from build123d import *

# Parameters (mm, degrees)
SKETCH1_W                      = 152.4
SKETCH1_H                      = 101.6
BASE_FLANGE1_DEPTH             = 1.29032
EDGE_FLANGE1_STRIP_W           = 5.85978
EDGE_FLANGE1_STRIP_H           = 1.29032
EDGE_FLANGE1_STRIP_CUT_DEPTH   = 101.6
EDGE_FLANGE1_STRIP_2_W         = 5.85978
EDGE_FLANGE1_STRIP_2_H         = 1.29032
EDGE_FLANGE1_STRIP_CUT_2_DEPTH = 101.6
EDGE_FLANGE1_DEPTH             = 101.6
EDGE_FLANGE1_BEND_DEPTH        = 101.6
M3X0_5_TAPPED_HOLE1_REACH      = 172.432
M3X0_5_TAPPED_HOLE1_BORE_R     = 1.5
BREAK_CORNER1_START            = -77.68082
BREAK_CORNER1_DEPTH            = 155.36164
CUT_THICKEN1_START             = 48.26
CUT_THICKEN1_OUTLINE_W         = 0.127
CUT_THICKEN1_OUTLINE_H         = 1.29032
CUT_THICKEN1_DEPTH             = 2.54
CUT_THICKEN2_START             = 48.26
CUT_THICKEN2_OUTLINE_W         = 0.127
CUT_THICKEN2_OUTLINE_H         = 1.29032
CUT_THICKEN2_DEPTH             = 2.54
MIRROR7_START                  = 48.26
MIRROR7_COPY_1_SKETCH_W        = 0.127
MIRROR7_COPY_1_SKETCH_H        = 1.29032
MIRROR7_COPY_1_DEPTH           = 2.54
MIRROR7_COPY_2_SKETCH_W        = 0.127
MIRROR7_COPY_2_SKETCH_H        = 1.29032
MIRROR7_COPY_2_DEPTH           = 2.54
MOVE_FACE1_BY                  = 1.27
MOVE_FACE1_2_BY                = 1.27
MOVE_FACE1_3_BY                = 1.27
MOVE_FACE1_4_BY                = 1.27
EDGE_FLANGE2_STRIP_W           = 5.66928
EDGE_FLANGE2_STRIP_H           = 1.29032
EDGE_FLANGE2_STRIP_CUT_DEPTH   = 2.54
EDGE_FLANGE2_STRIP_2_W         = 5.66928
EDGE_FLANGE2_STRIP_2_H         = 1.29032
EDGE_FLANGE2_STRIP_CUT_2_DEPTH = 2.54
EDGE_FLANGE2_STRIP_3_W         = 5.66928
EDGE_FLANGE2_STRIP_3_H         = 1.29032
EDGE_FLANGE2_STRIP_CUT_3_DEPTH = 2.54
EDGE_FLANGE2_STRIP_4_W         = 5.66928
EDGE_FLANGE2_STRIP_4_H         = 1.29032
EDGE_FLANGE2_STRIP_CUT_4_DEPTH = 2.54
EDGE_FLANGE2_DEPTH             = 2.54
EDGE_FLANGE2_BEND_DEPTH        = 2.54
EDGE_FLANGE2_BEND_2_DEPTH      = 2.54
EDGE_FLANGE2_BEND_3_DEPTH      = 2.54


# Read off the part's stored shape, not the designer's step: Break-Corner1, Cut-Thicken1, Cut-Thicken2
# Sheet-metal steps are written as plain solids
with BuildPart() as part:
    # Sketch1 → Base-Flange1 (new body)
    with BuildSketch(Plane.XY):
        Rectangle(SKETCH1_W, SKETCH1_H)
    extrude(amount=-BASE_FLANGE1_DEPTH)

    # Edge-Flange1 strip (across the edge) → Edge-Flange1 strip cut (cut)
    with BuildSketch(Plane(origin=(-76.3905, -50.8, -1.29032), x_dir=(1, 0, 0), z_dir=(0, 1, 0))):
        with Locations((-2.67589, -0.64516)):
            Rectangle(EDGE_FLANGE1_STRIP_W, EDGE_FLANGE1_STRIP_H)
    extrude(amount=EDGE_FLANGE1_STRIP_CUT_DEPTH, mode=Mode.SUBTRACT)

    # Edge-Flange1 strip 2 (across the edge) → Edge-Flange1 strip cut 2 (cut)
    with BuildSketch(Plane(origin=(76.3905, 50.8, -1.29032), x_dir=(-1, 0, 0), z_dir=(0, -1, 0))):
        with Locations((-2.67589, -0.64516)):
            Rectangle(EDGE_FLANGE1_STRIP_2_W, EDGE_FLANGE1_STRIP_2_H)
    extrude(amount=EDGE_FLANGE1_STRIP_CUT_2_DEPTH, mode=Mode.SUBTRACT)

    # Edge-Flange1 section (across the edge) → Edge-Flange1 (add)
    with BuildSketch(Plane(origin=(-76.3905, -50.8, -1.29032), x_dir=(1, 0, 0), z_dir=(0, 1, 0))):
        with BuildLine():
            Line((-1.29032, 0.254), (-1.29032, 46.96968))
            Line((-1.29032, 46.96968), (0, 46.96968))
            Line((0, 46.96968), (0, 0.254))
            ThreePointArc((0, 0.254), (0.074394878, 0.074394878), (0.254, 0))
            Line((0.254, 0), (0.254, -1.29032))
            ThreePointArc((0.254, -1.29032), (-0.837999144, -0.837999144), (-1.29032, 0.254))
        make_face()
    extrude(amount=EDGE_FLANGE1_DEPTH)

    # Edge-Flange1 section 2 (across the edge) → Edge-Flange1 bend (add)
    with BuildSketch(Plane(origin=(76.3905, 50.8, -1.29032), x_dir=(-1, 0, 0), z_dir=(0, -1, 0))):
        with BuildLine():
            Line((-1.29032, 0.254), (-1.29032, 46.96968))
            Line((-1.29032, 46.96968), (0, 46.96968))
            Line((0, 46.96968), (0, 0.254))
            ThreePointArc((0, 0.254), (0.074394878, 0.074394878), (0.254, 0))
            Line((0.254, 0), (0.254, -1.29032))
            ThreePointArc((0.254, -1.29032), (-0.837999144, -0.837999144), (-1.29032, 0.254))
        make_face()
    extrude(amount=EDGE_FLANGE1_BEND_DEPTH)

    # M3x0.5 Tapped Hole1 bore → M3x0.5 Tapped Hole1 (cut, up to next)
    with BuildSketch(Plane.ZY.offset(77.68082), mode=Mode.PRIVATE) as m3x0_5_tapped_hole1_sk1:
        with Locations((-44.7675, 0)):
            Circle(M3X0_5_TAPPED_HOLE1_BORE_R)
    m3x0_5_tapped_hole1_tool1 = extrude(m3x0_5_tapped_hole1_sk1.sketch, amount=-M3X0_5_TAPPED_HOLE1_REACH, mode=Mode.PRIVATE) & part.part
    m3x0_5_tapped_hole1 = m3x0_5_tapped_hole1_tool1.solids().sort_by_distance((-77.68082, 0, -44.7675))[0]
    add(m3x0_5_tapped_hole1, mode=Mode.SUBTRACT)

    # Mirror1: M3x0.5 Tapped Hole1 across plane
    add(m3x0_5_tapped_hole1.mirror(Plane(origin=(0, 0, 0), x_dir=(0, 0, 1), z_dir=(1, 0, 0))), mode=Mode.SUBTRACT)

    # Break-Corner1 outline → Break-Corner1 (cut)
    with BuildSketch(Plane.YZ.offset(BREAK_CORNER1_START)):
        with BuildLine():
            Line((50.8, -48.26), (50.8, -48.006))
            ThreePointArc((50.8, -48.006), (50.725605122, -48.185605122), (50.546, -48.26))
            Line((50.546, -48.26), (50.8, -48.26))
        make_face()
        with BuildLine():
            Line((-50.8, -48.26), (-50.546, -48.26))
            ThreePointArc((-50.546, -48.26), (-50.725605122, -48.185605122), (-50.8, -48.006))
            Line((-50.8, -48.006), (-50.8, -48.26))
        make_face()
    extrude(amount=BREAK_CORNER1_DEPTH, mode=Mode.SUBTRACT)

    # Cut-Thicken1 outline → Cut-Thicken1 (cut)
    with BuildSketch(Plane(origin=(0, 0, 0), x_dir=(1, 0, 0), z_dir=(0, 1, 0)).offset(CUT_THICKEN1_START)):
        with Locations((36.97732, 0.64516)):
            Rectangle(CUT_THICKEN1_OUTLINE_W, CUT_THICKEN1_OUTLINE_H)
    cut_thicken1 = extrude(amount=CUT_THICKEN1_DEPTH, mode=Mode.SUBTRACT)

    # Cut-Thicken2 outline → Cut-Thicken2 (cut)
    with BuildSketch(Plane(origin=(0, 0, 0), x_dir=(1, 0, 0), z_dir=(0, 1, 0)).offset(CUT_THICKEN2_START)):
        with Locations((39.64432, 0.64516)):
            Rectangle(CUT_THICKEN2_OUTLINE_W, CUT_THICKEN2_OUTLINE_H)
    cut_thicken2 = extrude(amount=CUT_THICKEN2_DEPTH, mode=Mode.SUBTRACT)

    # Mirror6: Cut-Thicken1, Cut-Thicken2 across plane
    add(cut_thicken1.mirror(Plane(origin=(0, 0, 0), x_dir=(0, 0, 1), z_dir=(1, 0, 0))), mode=Mode.SUBTRACT)
    add(cut_thicken2.mirror(Plane(origin=(0, 0, 0), x_dir=(0, 0, 1), z_dir=(1, 0, 0))), mode=Mode.SUBTRACT)

    # Mirror7: Cut-Thicken1, Cut-Thicken2 across plane
    add(cut_thicken1.mirror(Plane.ZX), mode=Mode.SUBTRACT)
    add(cut_thicken2.mirror(Plane.ZX), mode=Mode.SUBTRACT)

    # Mirror7 copy 1 sketch → Mirror7 copy 1 (cut)
    with BuildSketch(Plane(origin=(0, 0, 0), x_dir=(-1, 0, 0), z_dir=(0, -1, 0)).offset(MIRROR7_START)):
        with Locations((36.97732, 0.64516)):
            Rectangle(MIRROR7_COPY_1_SKETCH_W, MIRROR7_COPY_1_SKETCH_H)
    extrude(amount=MIRROR7_COPY_1_DEPTH, mode=Mode.SUBTRACT)

    # Mirror7 copy 2 sketch → Mirror7 copy 2 (cut)
    with BuildSketch(Plane(origin=(0, 0, 0), x_dir=(-1, 0, 0), z_dir=(0, -1, 0)).offset(MIRROR7_START)):
        with Locations((39.64432, 0.64516)):
            Rectangle(MIRROR7_COPY_2_SKETCH_W, MIRROR7_COPY_2_SKETCH_H)
    extrude(amount=MIRROR7_COPY_2_DEPTH, mode=Mode.SUBTRACT)

    # Move Face1: a face moved inward by 1.27
    extrude(part.faces().sort_by_distance((-38.31082, -50.8, -0.64516))[0], amount=MOVE_FACE1_BY, dir=(0, 1, 0), mode=Mode.SUBTRACT)

    # Move Face1 2: a face moved inward by 1.27
    extrude(part.faces().sort_by_distance((38.31082, -50.8, -0.64516))[0], amount=MOVE_FACE1_2_BY, dir=(0, 1, 0), mode=Mode.SUBTRACT)

    # Move Face1 3: a face moved inward by 1.27
    extrude(part.faces().sort_by_distance((-38.31082, 50.8, -0.64516))[0], amount=MOVE_FACE1_3_BY, dir=(0, -1, 0), mode=Mode.SUBTRACT)

    # Move Face1 4: a face moved inward by 1.27
    extrude(part.faces().sort_by_distance((38.31082, 50.8, -0.64516))[0], amount=MOVE_FACE1_4_BY, dir=(0, -1, 0), mode=Mode.SUBTRACT)

    # Edge-Flange2 strip (across the edge) → Edge-Flange2 strip cut (cut)
    with BuildSketch(Plane(origin=(37.04082, 49.53, -1.29032), x_dir=(0, -1, 0), z_dir=(1, 0, 0))):
        with Locations((-1.29032, -0.64516)):
            Rectangle(EDGE_FLANGE2_STRIP_W, EDGE_FLANGE2_STRIP_H)
    extrude(amount=EDGE_FLANGE2_STRIP_CUT_DEPTH, mode=Mode.SUBTRACT)

    # Edge-Flange2 strip 2 (across the edge) → Edge-Flange2 strip cut 2 (cut)
    with BuildSketch(Plane(origin=(-39.58082, 49.53, -1.29032), x_dir=(0, -1, 0), z_dir=(1, 0, 0))):
        with Locations((-1.29032, -0.64516)):
            Rectangle(EDGE_FLANGE2_STRIP_2_W, EDGE_FLANGE2_STRIP_2_H)
    extrude(amount=EDGE_FLANGE2_STRIP_CUT_2_DEPTH, mode=Mode.SUBTRACT)

    # Edge-Flange2 strip 3 (across the edge) → Edge-Flange2 strip cut 3 (cut)
    with BuildSketch(Plane(origin=(39.58082, -49.53, -1.29032), x_dir=(0, 1, 0), z_dir=(-1, 0, 0))):
        with Locations((-1.29032, -0.64516)):
            Rectangle(EDGE_FLANGE2_STRIP_3_W, EDGE_FLANGE2_STRIP_3_H)
    extrude(amount=EDGE_FLANGE2_STRIP_CUT_3_DEPTH, mode=Mode.SUBTRACT)

    # Edge-Flange2 strip 4 (across the edge) → Edge-Flange2 strip cut 4 (cut)
    with BuildSketch(Plane(origin=(-37.04082, -49.53, -1.29032), x_dir=(0, 1, 0), z_dir=(-1, 0, 0))):
        with Locations((-1.29032, -0.64516)):
            Rectangle(EDGE_FLANGE2_STRIP_4_W, EDGE_FLANGE2_STRIP_4_H)
    extrude(amount=EDGE_FLANGE2_STRIP_CUT_4_DEPTH, mode=Mode.SUBTRACT)

    # Edge-Flange2 section (across the edge) → Edge-Flange2 (add)
    with BuildSketch(Plane(origin=(37.04082, 49.53, -1.29032), x_dir=(0, -1, 0), z_dir=(1, 0, 0))):
        with BuildLine():
            Line((0, 0.254), (0, 1.27))
            Line((0, 1.27), (1.29032, 1.27))
            Line((1.29032, 1.27), (1.29032, 0.254))
            ThreePointArc((1.29032, 0.254), (1.364714878, 0.074394878), (1.54432, 0))
            Line((1.54432, 0), (1.54432, -1.29032))
            ThreePointArc((1.54432, -1.29032), (0.452320856, -0.837999144), (0, 0.254))
        make_face()
    extrude(amount=EDGE_FLANGE2_DEPTH)

    # Edge-Flange2 section 2 (across the edge) → Edge-Flange2 bend (add)
    with BuildSketch(Plane(origin=(-39.58082, 49.53, -1.29032), x_dir=(0, -1, 0), z_dir=(1, 0, 0))):
        with BuildLine():
            Line((0, 0.254), (0, 1.27))
            Line((0, 1.27), (1.29032, 1.27))
            Line((1.29032, 1.27), (1.29032, 0.254))
            ThreePointArc((1.29032, 0.254), (1.364714878, 0.074394878), (1.54432, 0))
            Line((1.54432, 0), (1.54432, -1.29032))
            ThreePointArc((1.54432, -1.29032), (0.452320856, -0.837999144), (0, 0.254))
        make_face()
    extrude(amount=EDGE_FLANGE2_BEND_DEPTH)

    # Edge-Flange2 section 3 (across the edge) → Edge-Flange2 bend 2 (add)
    with BuildSketch(Plane(origin=(39.58082, -49.53, -1.29032), x_dir=(0, 1, 0), z_dir=(-1, 0, 0))):
        with BuildLine():
            Line((0, 0.254), (0, 1.27))
            Line((0, 1.27), (1.29032, 1.27))
            Line((1.29032, 1.27), (1.29032, 0.254))
            ThreePointArc((1.29032, 0.254), (1.364714878, 0.074394878), (1.54432, 0))
            Line((1.54432, 0), (1.54432, -1.29032))
            ThreePointArc((1.54432, -1.29032), (0.452320856, -0.837999144), (0, 0.254))
        make_face()
    extrude(amount=EDGE_FLANGE2_BEND_2_DEPTH)

    # Edge-Flange2 section 4 (across the edge) → Edge-Flange2 bend 3 (add)
    with BuildSketch(Plane(origin=(-37.04082, -49.53, -1.29032), x_dir=(0, 1, 0), z_dir=(-1, 0, 0))):
        with BuildLine():
            Line((0, 0.254), (0, 1.27))
            Line((0, 1.27), (1.29032, 1.27))
            Line((1.29032, 1.27), (1.29032, 0.254))
            ThreePointArc((1.29032, 0.254), (1.364714878, 0.074394878), (1.54432, 0))
            Line((1.54432, 0), (1.54432, -1.29032))
            ThreePointArc((1.54432, -1.29032), (0.452320856, -0.837999144), (0, 0.254))
        make_face()
    extrude(amount=EDGE_FLANGE2_BEND_3_DEPTH)


solid = part.part
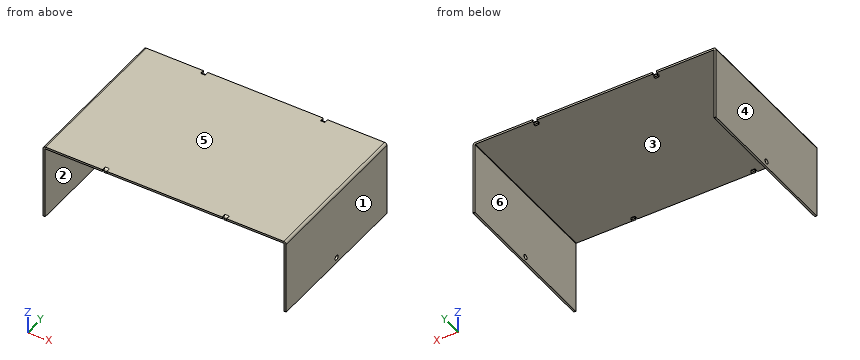
Read the model definition and answer for the solid it produces. Units are mm, in the model's axes. Face numbers are marked on the shaded views. A direction names the side the tool comes from. Round coordinates to 2 decimals unless told otherwise and drop trailing zeros. Write each loop counter-clockwise with the first axis right and the second up, starting at its lowest first coordinate (ties: lowest second). Pieces come first, ordered by that corner, then holes. Notation, with made-up numbers: (46, 22) - (99, 22) arc R13 ccw to (99, 37) - close; hole circle Ø4 at (-15.5, 28.5). An arc over 180 degrees is marked (long way). One line per question, with ' | ' between items. Start each with the question number.
1. Section A-A (z = -13) is taken. Determine the outline of the cut face in (x, y).
2. Section C-C (x = 68) is taken. Determine the outline of the cut face in (y, z).
3. Section B-B (y = 35.5) is taken. Determine the outline of the cut face in (x, z), and give its area (3 significant figures).
4. For the marked faces 5 and 6, determine the directions among +Z, -Z, +X, -X, +Y, -Y from which every point of the face is accessible in a straight line to the end or side of a thin tool.
5. Find the intervals of material crossed by probe 1 along X at (y, z) = (-38.5, -14); probe 2 along Z at (x, y) = (25, 12), in increasing order. Write a range as [from, to].
6. For a pull along X with two mould halves and no side action, classify the marked faces 1, 2, 3 and 4 as +X half, -X half, draft (parallel to the pull), parting line (faces both ways), or undercut.
7. Each of these flat-tipped pins is pushed along its axis until it touches: pin 1 (0.6 mm diameter, centred on y = 49.5, z = -0.5, fed in from +X); pin 2 (3 mm diameter, centred on x = 20, y = -2.5, fed in from +Z); pin 3 (2 mm diameter, centred on x = -18.5, y = 15, fed in from -Z); pin 4 (1.1 mm diameter, centred on x = 38, z = -2, fed in from -Y). Where does it stop, or does it pass through?
Filled in:
1) outline: (-77.68, -50.8) - (-76.39, -50.8) - (-76.39, 50.8) - (-77.68, 50.8) - close; (76.39, -50.8) - (77.68, -50.8) - (77.68, 50.8) - (76.39, 50.8) - close
2) outline: (-50.8, -1.29) - (50.8, -1.29) - (50.8, 0) - (-50.8, 0) - close
3) outline: (-77.68, -48.26) - (-76.39, -48.26) - (-76.39, -1.54) arc R0.25 cw to (-76.14, -1.29) - (76.14, -1.29) arc R0.25 cw to (76.39, -1.54) - (76.39, -48.26) - (77.68, -48.26) - (77.68, -1.54) arc R1.54 ccw to (76.14, 0) - (-76.14, 0) arc R1.54 ccw to (-77.68, -1.54) - close | area: 321 mm²
4) face 5: +Z, +X, -X, +Y, -Y | face 6: -Z, +Y, -Y
5) probe 1: [-77.68, -76.39], [76.39, 77.68] | probe 2: [-1.29, 0]
6) face 1: +X half | face 2: undercut | face 3: undercut | face 4: -X half
7) pin 1: x = 77.49 | pin 2: z = 0 | pin 3: z = -1.29 | pin 4: y = -49.53
